Design review of the part shown in the three views and the two pictorial views. Dimensions are in mm from the part's minimum x, y and z. Coordinates: 2 decimals unless noted, no trailing zeros. Loops run counter-clockwise (first coordinate to the right, second up) from the corner with the lowest first, then second, coordinate; pieces in that order, holes last. Notation, with made-up numbers: (1.25, 11.25) -> (30.25, 11.25) arc R13 cw to (30.25, 30.25) -> close; hole circle Ø3 at (-12.75, 4.5). An arc over 180 degrees is marked (long way). Answer in a Markdown table with one row per item.
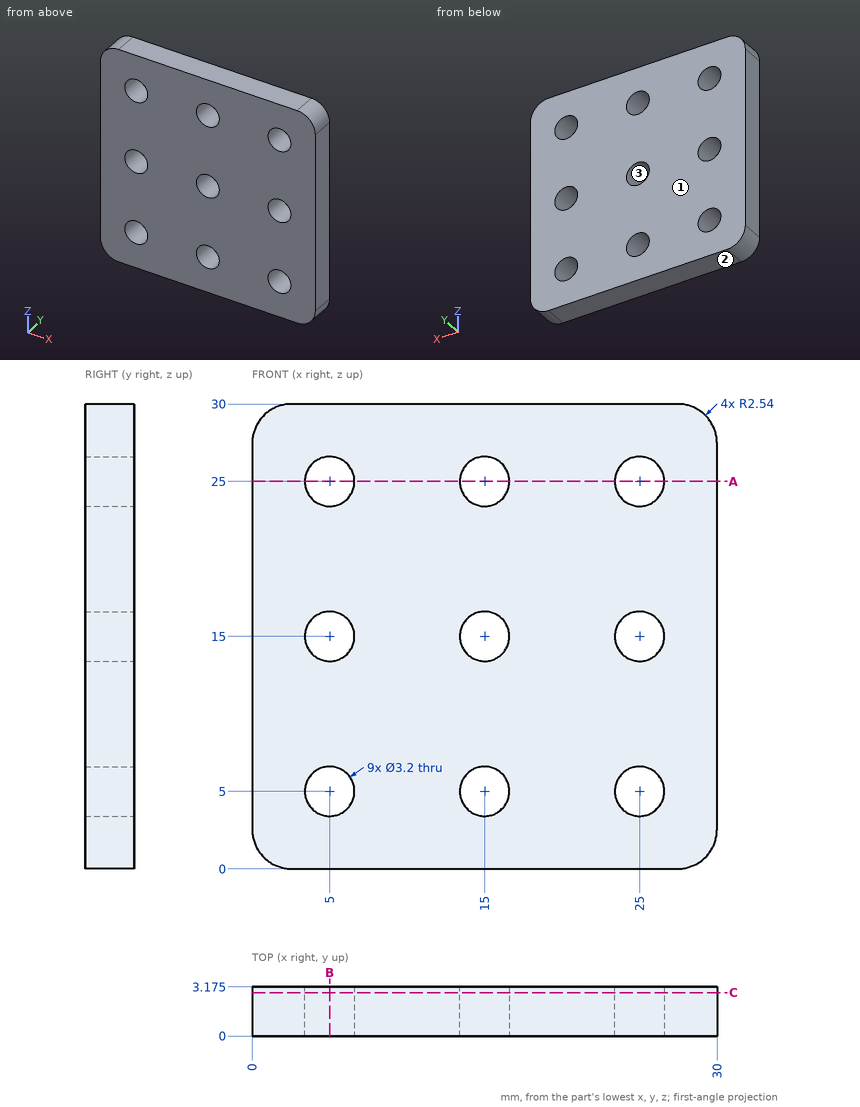
(1) Draft analysis for pull direction Z (two halves, no side actions). For the marked faces 1, 2 and 3, state which applies: pulls with the +Z half, pulls with the -Z half, needs draft (parallel to the pull), parting line crosses it, or undercut.
Evaluation:
| item | result |
|---|---|
| face 1 | needs draft |
| face 2 | pulls with the -Z half |
| face 3 | undercut |
(2) To check wall thickness, follow probe 1 along Z at (x, y) = (5, 2.1); probe 2 along Z at (x, y) = (16, 2.1); probe 3 along X at (y, z) = (1.5, 25.5). State the ranges of each line that lie inside material, in increasing order.
Evaluation:
| item | result |
|---|---|
| probe 1 | z = 0 to 3.4, 6.6 to 13.4, 16.6 to 23.4, 26.6 to 30 |
| probe 2 | z = 0 to 3.75, 6.25 to 13.75, 16.25 to 23.75, 26.25 to 30 |
| probe 3 | x = 0 to 3.48, 6.52 to 13.48, 16.52 to 23.48, 26.52 to 30 |
(3) Take a section at A-A on z = 25. Give the boundary of the cut face in (x, y) (3 decimals), and give its area (3 significant figures).
Evaluation:
| item | result |
|---|---|
| outline | (0, 0) -> (3.4, 0) -> (3.4, 3.175) -> (0, 3.175) -> close; (6.6, 0) -> (13.4, 0) -> (13.4, 3.175) -> (6.6, 3.175) -> close; (16.6, 0) -> (23.4, 0) -> (23.4, 3.175) -> (16.6, 3.175) -> close; (26.6, 0) -> (30, 0) -> (30, 3.175) -> (26.6, 3.175) -> close |
| area | 64.8 mm² |
(4) Take a section at B-B on x = 5. Give the boundary of the cut face in (y, z) (3 decimals), and give its area (3 significant figures).
Evaluation:
| item | result |
|---|---|
| outline | (0, 0) -> (3.175, 0) -> (3.175, 3.4) -> (0, 3.4) -> close; (0, 6.6) -> (3.175, 6.6) -> (3.175, 13.4) -> (0, 13.4) -> close; (0, 16.6) -> (3.175, 16.6) -> (3.175, 23.4) -> (0, 23.4) -> close; (0, 26.6) -> (3.175, 26.6) -> (3.175, 30) -> (0, 30) -> close |
| area | 64.8 mm² |
(5) Take a section at C-C on y = 2.8. Count the separate pieces of the cut face and the enclosed holes in it, and give its area (3 significant figures).
Evaluation:
| item | result |
|---|---|
| separate pieces | 1 |
| enclosed holes | 9 |
| area | 822 mm² |
(6) For pin 1 (3 mm diameter, centred on x = 25, z = 5, fed in from +Y), flat-tipped, find the tip position at first contact; note if it passes through.
Evaluation:
| item | result |
|---|---|
| pin 1 | passes through |
